Input: part model. Units: mm. Frame: model coordinates. A direction names the side the tool comes from. Give positions to 0.01 mm unless a question says otherwise; leave off trailing zeros. Loops run counter-clockwise (first coordinate to the right, second up) from the corner with the lowest first, then second, coordinate; pieces in that order, holes last. Notation, with made-up numbers: (59.25, 75.5) - (107.25, 75.5) arc R13 cw to (107.25, 86.5) - close; hole circle Ø10 at (15, 16.5). An arc over 180 degrees is marked (long way). Answer as a JSON object with one key per item and string values.
Autodesk Inventor part; units mm, degrees
ref_plane "YZ Plane" through (0, 0, 0) normal (1, 0, 0) x (0, 1, 0)
ref_plane "XZ Plane" through (0, 0, 0) normal (0, 1, 0) x (-1, 0, 0)
ref_plane "XY Plane" through (0, 0, 0) normal (0, 0, 1) x (1, 0, 0)
sketch "Sketch1" plane through (0, 0, 0) normal (0, 1, 0) x (-1, 0, 0)
  circle A0 centre (0, 0) radius 11.938 construction
  line L0 (0, 0) -> (-54.7943, -30.1916) construction
  line L1 (0, 0) -> (-11.938, 0) construction
  circle A1 centre (-54.7943, -30.1916) radius 11.938 construction
  line L2 (-49.0331, -40.6475) -> (5.7612, -10.4559)
  line L3 (-60.5554, -19.7358) -> (-5.7612, 10.4559)
  arc A2 (-60.5554, -19.7358) -> (-49.0331, -40.6475) centre (-54.7943, -30.1916) ccw
  arc A3 (5.7612, -10.4559) -> (-5.7612, 10.4559) centre (0, 0) ccw
  line L4 (-6.9869, 12.6805) -> (-61.7812, -17.5111)
  arc A4 (-61.7812, -17.5111) -> (-47.8073, -42.8721) centre (-54.7943, -30.1916) ccw
  line L5 (-47.8073, -42.8721) -> (6.9869, -12.6805)
  arc A5 (6.9869, -12.6805) -> (-6.9869, 12.6805) centre (0, 0) ccw
  dimension "d11" = 23.876
  dimension "d12" = 28.855
  dimension "d13" = 62.5615
  dimension "d14" = 2.54
extrude "Extrusion2" add sketch "Sketch1" along normal blind 8.9916
properties part number "INtk_010_Belt2" material "Rubber, Silicone"
Item 1: Material intervals for line 1 (Z direction, x = 19.5, y = 8.25); line 2 (X direction, y = 6.25, z = -27); line 3 (Z direction, x = 6, y = 7), sorted ascending. Write a range as [from, to].
Geometry check:
{"line 1": "z = [-27.27, -24.37], [2.89, 5.79]", "line 2": "x = [19, 24.26], [66.3, 68.92]", "line 3": "z = [-19.84, -16.94], [10.32, 13.18]"}
Item 2: Cut plane B-B (x = 0). Return loops of the section in (y, z).
Geometry check:
{"outline": "(0, -16.53) - (8.99, -16.53) - (8.99, -13.63) - (0, -13.63) - close; (0, 11.94) - (8.99, 11.94) - (8.99, 14.48) - (0, 14.48) - close"}
Item 3: Cut plane A-A (z = -38). Return loops of the section in (x, y), then the cut area to 3 significant figures.
Geometry check:
{"outline": "(38.97, 0) - (44.23, 0) - (44.23, 8.99) - (38.97, 8.99) - close; (63.82, 0) - (66.99, 0) - (66.99, 8.99) - (63.82, 8.99) - close", "area": "75.8 mm2"}
Item 4: Mould query, pull axis Z, two halves, no side actions, for faces 3 (the face through (67.318, 4.433, -37.456)), 4 (the face through (20.794, 4.433, -27.988)), 5 (the face through (21, 0, -26)), 6 (the face through (22.02, 4.433, -25.763)). Classes: released by +Z, released by -Z, zero draft, split by the parting line, or undercut.
Geometry check:
{"face 3": "split by the parting line", "face 4": "released by -Z", "face 5": "zero draft", "face 6": "undercut"}
Item 5: Access query for faces 1 (the face through (34, 4.433, -2.204)), 2 (the face through (33.54, 4.43, -4.85)). Directions: +Z, -Z, +X, -X, +Y, -Y. A direction counts if a zero-diameter tool reaches every point of the face in a straight line with its end or side. Return the directions, or none.
Geometry check:
{"face 1": "+Z, +X, +Y, -Y", "face 2": "+Y, -Y"}
Item 6: Contact query for flat-ended pins moving along their axis: P1, Ø4, axis at x = 33.5, y = 5, coming from the -Z side; P2, Ø3, axis at y = 7.5, z = -5.5, coming from the -X side; P3, Ø3, axis at x = 23, y = 3.5, coming from the -Z side. Output: stop coordinate, or through.
Geometry check:
{"P1": "stops at z = -36.09", "P2": "stops at x = -13.91", "P3": "stops at z = -30.03"}
